Source: CAD feature listing. Evaluate the final solid. Frame: model axes, mm. Give positions to 0.01 mm unless a question says otherwise; leave off trailing zeros. Loops run counter-clockwise (first coordinate to the right, second up) from the corner with the lowest first, then second, coordinate; pieces in that order, holes last. Notation, with made-up numbers: (-31, -38) -> (-11, -38) arc R23 ccw to (-11, -2) -> close; hole circle Ø6 at (45, 44.5). An arc over 180 degrees is marked (long way). Answer as a JSON object with one key per item and string values. Group by question number.
from build123d import *

# Parameters (mm, degrees)
SKETCH1_W           = 181
SKETCH1_H           = 75.57
BOSS_EXTRUDE2_DEPTH = 4.75
SKETCH6_W           = 3
SKETCH6_H           = 10
SKETCH6_W_2         = 10
SKETCH6_H_2         = 2.996296141
SKETCH6_W_3         = 9.939831887
SKETCH6_H_3         = 3
SKETCH6_W_4         = 20
SKETCH6_H_4         = 41
SKETCH6_R           = 1.75
SKETCH6_R_2         = 1.25
CUT_EXTRUDE7_DEPTH  = 9


with BuildPart() as part:
    # Sketch1 → Boss-Extrude2 (new body)
    with BuildSketch(Plane.XY):
        Rectangle(SKETCH1_W, SKETCH1_H)
    extrude(amount=BOSS_EXTRUDE2_DEPTH)

    # Sketch6 → Cut-Extrude7 (cut)
    with BuildSketch(Plane.XY.offset(4.75)):
        with BuildLine():
            Line((-90.5, 37.785), (-90.5, 35.274795088))
            ThreePointArc((-90.5, 35.274795088), (-89.587457665, 37.010103297), (-87.786468161, 37.785))
            Line((-87.786468161, 37.785), (-90.5, 37.785))
        make_face()
        with BuildLine():
            ThreePointArc((-87.786468161, -37.785), (-89.587457665, -37.010103297), (-90.5, -35.274795088))
            Line((-90.5, -35.274795088), (-90.5, -37.785))
            Line((-90.5, -37.785), (-87.786468161, -37.785))
        make_face()
        Polygon((90.5, 37.785), (38.141923512, 37.785), (61.552812751, 32.14), (90.5, 17.2), align=None)
        Polygon((61.552812751, -32.135214744), (38.141923512, -37.785), (90.5, -37.785), (90.5, -17.2), align=None)
        Polygon((-81.947178372, 35.785), (-81.913405317, 32.785953243), (-71.879658735, 32.785762546), (-71.94729523, 35.785), align=None)
        with Locations((-88, 18.75)):
            Rectangle(SKETCH6_W, SKETCH6_H)
        with Locations((-88, -18.75)):
            Rectangle(SKETCH6_W, SKETCH6_H)
        Polygon((-33.930858677, 35.785), (-33.929672617, 32.785000234), (-23.927298062, 32.788706115), (-23.930975535, 35.785), align=None)
        Polygon((-71.879658735, -32.785190697), (-81.913405317, -32.785000001), (-81.913478974, -35.785), (-71.913483982, -35.785), align=None)
        Polygon((-33.903748919, -32.785912448), (-33.902562858, -35.785912214), (-23.88684069, -35.786102825), (-23.88684069, -32.786102825), align=None)
        with Locations((87, 9.9)):
            Rectangle(SKETCH6_W, SKETCH6_H)
        with Locations((24.052991197, 34.28685193)):
            Rectangle(SKETCH6_W_2, SKETCH6_H_2)
        with Locations((24.083075253, -34.285)):
            Rectangle(SKETCH6_W_3, SKETCH6_H_3)
        with Locations((-4.459374015, 0.957016564)):
            Rectangle(SKETCH6_W_4, SKETCH6_H_4)
        with Locations((87, -9.9)):
            Rectangle(SKETCH6_W, SKETCH6_H)
        with Locations((-9.629374015, 25.857016564)):
            Circle(SKETCH6_R)
        with Locations((0.370625985, 25.857016564)):
            Circle(SKETCH6_R)
        with Locations((0.370625985, -23.942983436)):
            Circle(SKETCH6_R)
        with Locations((-9.629374015, -23.942983436)):
            Circle(SKETCH6_R)
        with Locations((11.052985258, -29)):
            Circle(SKETCH6_R)
        with Locations((11.052985258, 29)):
            Circle(SKETCH6_R)
        with Locations((60.052985258, -29)):
            Circle(SKETCH6_R)
        with Locations((60.052985258, 29)):
            Circle(SKETCH6_R)
        with Locations((-79.373192673, 24.5)):
            Circle(SKETCH6_R_2)
        with Locations((-79.373192673, -24.5)):
            Circle(SKETCH6_R_2)
        with Locations((-21.373192673, -24.5)):
            Circle(SKETCH6_R_2)
        with Locations((-21.373192673, 24.5)):
            Circle(SKETCH6_R_2)
    extrude(amount=-CUT_EXTRUDE7_DEPTH, mode=Mode.SUBTRACT)


solid = part.part
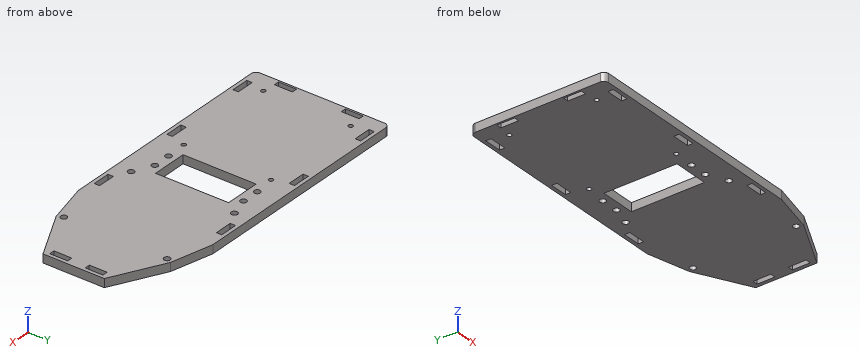
(1) Section query A-A on y = 9. Return the cut outline in (x, z).
(2) Material intervals for line 1 (X direction, y = -5, z = 0.85); line 2 (X direction, y = -15.5, z = 3.6); line 3 (Y direction, x = -29, z = 0.3) (3 decimals), sorted ascending. Write a range as from..to.
(3) Section query D-D on x = 50. Return the cut outline in (y, z), plus the area to 3 significant figures.
(4) Section query B-B on x = -29. Return the cut outline in (y, z) (3 decimals).
(5) Section query C-C on z = 1.85. State how many separate pieces and enclosed holes the cut face has, plus the area to 3 significant figures.
Result:
{
 "1": {"outline": "(-90.5, 0) -> (-14.46, 0) -> (-14.46, 4.75) -> (-90.5, 4.75) -> close; (5.54, 0) -> (85.5, 0) -> (85.5, 4.75) -> (5.54, 4.75) -> close; (88.5, 0) -> (90.5, 0) -> (90.5, 4.75) -> (88.5, 4.75) -> close"},
 "2": {"line 1": "-90.5..-14.46, 5.54..85.5, 88.5..90.5", "line 2": "-90.5..-89.5, -86.5..-14.46, 5.54..90.5", "line 3": "-37.785..-35.786, -32.786..32.787, 35.785..37.785"},
 "3": {"outline": "(-34.92, 0) -> (34.93, 0) -> (34.93, 4.75) -> (-34.92, 4.75) -> close", "area": "332 mm²"},
 "4": {"outline": "(-37.785, 0) -> (-35.786, 0) -> (-35.786, 4.75) -> (-37.785, 4.75) -> close; (-32.786, 0) -> (32.787, 0) -> (32.787, 4.75) -> (-32.786, 4.75) -> close; (35.785, 0) -> (37.785, 0) -> (37.785, 4.75) -> (35.785, 4.75) -> close"},
 "5": {"separate pieces": "1", "enclosed holes": "23", "area": "11,600 mm²"}
}
